```python
from build123d import *

# Parameters (mm, degrees)
F0_W     = 76.2
F0_H     = 25.4
F0_R     = 1.85
F0_R_2   = 4
F1_DEPTH = 5.08
F2_W     = 7.62
F2_H     = 25.4
F3_DEPTH = 25.4
F4_W     = 12.7
F4_H     = 25.4
F4_R     = 1.85
F4_W_2   = 7.62
F4_W_3   = 20.32
F5_DEPTH = 3.175


with BuildPart() as f1:
    # F0 (on Top) → F1 (new body)
    with BuildSketch(Plane.XY):
        Rectangle(F0_W, F0_H)
        with Locations((-5.656854, -5.656854)):
            Circle(F0_R, mode=Mode.SUBTRACT)
        with Locations((-8, 0)):
            Circle(F0_R, mode=Mode.SUBTRACT)
        with Locations((0, -8)):
            Circle(F0_R, mode=Mode.SUBTRACT)
        with Locations((5.656854, -5.656854)):
            Circle(F0_R, mode=Mode.SUBTRACT)
        Circle(F0_R_2, mode=Mode.SUBTRACT)
        with Locations((8, 0)):
            Circle(F0_R, mode=Mode.SUBTRACT)
        with Locations((-5.656854, 5.656854)):
            Circle(F0_R, mode=Mode.SUBTRACT)
        with Locations((5.656854, 5.656854)):
            Circle(F0_R, mode=Mode.SUBTRACT)
        with Locations((0, 8)):
            Circle(F0_R, mode=Mode.SUBTRACT)
    extrude(amount=F1_DEPTH)

    # F2 (on face) → F3 (join)
    with BuildSketch(Plane(origin=(0, 0, 0), x_dir=(1, 0, 0), z_dir=(0, 0, -1))):
        with Locations((34.29, 0)):
            Rectangle(F2_W, F2_H)
        with Locations((-34.29, 0)):
            Rectangle(F2_W, F2_H)
    extrude(amount=F3_DEPTH)

    # F4 (on face) → F5 (join)
    with BuildSketch(Plane(origin=(0, 0, -25.4), x_dir=(1, 0, 0), z_dir=(0, 0, -1))):
        with Locations((-44.45, 0)):
            Rectangle(F4_W, F4_H)
        with Locations((-44.45, -6.35)):
            Circle(F4_R, mode=Mode.SUBTRACT)
        with Locations((-44.45, 6.35)):
            Circle(F4_R, mode=Mode.SUBTRACT)
        with Locations((-34.29, 0)):
            Rectangle(F4_W_2, F4_H)
        with Locations((40.64, 0)):
            Rectangle(F4_W_3, F4_H)
        with Locations((44.45, -6.35)):
            Circle(F4_R, mode=Mode.SUBTRACT)
        with Locations((44.45, 6.35)):
            Circle(F4_R, mode=Mode.SUBTRACT)
    extrude(amount=F5_DEPTH)


solid = f1.part
```
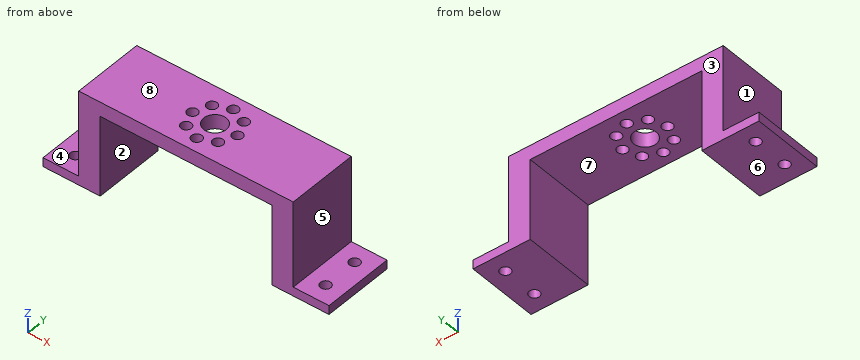
Check sheet for the modelled part. Datum: model origin and axes. Units: mm. Face numbers are marked on the shaded views. A direction names the side the tool comes from. Give positions to 0.01 mm unless a question says otherwise; leave off trailing zeros. Order: outer loops, then holes, each group sorted by start corner. A loop starts at its lowest first (then second) coordinate and runs counter-clockwise, first axis right, second up. Notation, with made-up numbers: M -23.75,13 L 24.25,13 A13 ccw 24.25,38 Z; hole C 46,82 d5. An arc over 180 degrees is marked long. Answer in a Markdown table with one row per item.
1) Release check for a two-part mould opening along X. For the marked faces 1, 2 and 3 record: +X half, -X half, draft (parallel to the pull), parting line (faces both ways), or undercut.
Filled sheet:
| item | result |
|---|---|
| face 1 | -X half |
| face 2 | undercut |
| face 3 | draft |
2) Cross-section at A-A, the plane z = -11.5. Enter the section's corners in (x, y), plus the area to 3 significant figures.
Filled sheet:
| item | result |
|---|---|
| outline | M -38.1,-12.7 L -30.48,-12.7 L -30.48,12.7 L -38.1,12.7 Z; M 30.48,-12.7 L 38.1,-12.7 L 38.1,12.7 L 30.48,12.7 Z |
| area | 387 mm2 |
3) Cross-section at C-C, the plane y = 2.75. Enter the section's corners in (x, z) (3 decimals), plus the area to 3 significant figures.
Filled sheet:
| item | result |
|---|---|
| outline | M -50.8,-28.575 L -30.48,-28.575 L -30.48,0 L -2.905,0 L -2.905,5.08 L -38.1,5.08 L -38.1,-25.4 L -50.8,-25.4 Z; M 2.905,0 L 30.48,0 L 30.48,-28.575 L 50.8,-28.575 L 50.8,-25.4 L 38.1,-25.4 L 38.1,5.08 L 2.905,5.08 Z |
| area | 874 mm2 |
4) Thickness scan on L1, parallel to X at y = -6.35, z = -27.75; L2, parallel to Y at x = -44.45, z = -27.25; L3, parallel to X at y = -6, z = -24. Record the ranges inside material, lowest first. Write a range as [from, to].
Filled sheet:
| item | result |
|---|---|
| L1 | x = [-50.8, -46.3], [-42.6, -30.48], [30.48, 42.6], [46.3, 50.8] |
| L2 | y = [-12.7, -8.2], [-4.5, 4.5], [8.2, 12.7] |
| L3 | x = [-38.1, -30.48], [30.48, 38.1] |
5) Gauge pin test, flat ends, axial feed: P1, Ø3.5, axis at x = 0, y = -8, coming from the -Z side; P2, Ø7.5, axis at x = 15, y = 2.5, coming from the -Z side; P3, Ø6.5, axis at x = -44, y = -3, coming from the +Z side; P4, Ø5, axis at x = -8, y = 0, coming from the +Z side. Record the tip position at first contact, or that the pin passes through.
Filled sheet:
| item | result |
|---|---|
| P1 | passes through |
| P2 | stops at z = 0 |
| P3 | stops at z = -25.4 |
| P4 | stops at z = 5.08 |
6) Cross-section at D-D, the plane x = 0. Enter the section's corners in (y, z), plus the area to 3 significant figures.
Filled sheet:
| item | result |
|---|---|
| outline | M -12.7,0 L -9.85,0 L -9.85,5.08 L -12.7,5.08 Z; M -6.15,0 L -4,0 L -4,5.08 L -6.15,5.08 Z; M 4,0 L 6.15,0 L 6.15,5.08 L 4,5.08 Z; M 9.85,0 L 12.7,0 L 12.7,5.08 L 9.85,5.08 Z |
| area | 50.8 mm2 |
7) Cross-section at B-B, the plane x = 44.45. Enter the section's corners in (y, z) (3 decimals), plus the area to 4 significant figures.
Filled sheet:
| item | result |
|---|---|
| outline | M -12.7,-28.575 L -8.2,-28.575 L -8.2,-25.4 L -12.7,-25.4 Z; M -4.5,-28.575 L 4.5,-28.575 L 4.5,-25.4 L -4.5,-25.4 Z; M 8.2,-28.575 L 12.7,-28.575 L 12.7,-25.4 L 8.2,-25.4 Z |
| area | 57.15 mm2 |
8) Access from +Z, -Z, +X, -X, +Y, -Y to the whole of each face (thin tool, end or side, straight path). Record for the marked faces 4, 5, 6, 7 and 8.
Filled sheet:
| item | result |
|---|---|
| face 4 | +Z, -X, +Y, -Y |
| face 5 | +Z, +X, +Y, -Y |
| face 6 | -Z, +X, -X, +Y, -Y |
| face 7 | -Z, +Y, -Y |
| face 8 | +Z, +X, -X, +Y, -Y |
